from build123d import *

# Parameters (mm, degrees)
ESBO_O2_R                  = 2.8
CORTE_EXTRUS_O1_DEPTH      = 10
CORTE_EXTRUS_O1_DEPTH_BACK = 10
RESSALTO_EXTRUS_O1_START   = -12
ESBO_O5_W                  = 5.6
ESBO_O5_H                  = 16
RESSALTO_EXTRUS_O1_DEPTH   = 80
FILETE1_R                  = 5
CORTE_EXTRUS_O2_DEPTH      = 19


with BuildPart() as part:
    # Esbo_o2 → Revolu_o1 (revolve)
    with BuildSketch(Plane(origin=(0, 0, 0), x_dir=(1, 0, 0), z_dir=(0, 1, 0))):
        with Locations((13.75, 0)):
            Circle(ESBO_O2_R)
    revolve(axis=Axis((0, 0, 0), (0, 0, -1)))

    # Esbo_o3 → Corte-extrus_o1 (cut, two sides)
    with BuildSketch(Plane.XY) as corte_extrus_o1_sk:
        Polygon((-1.202746457, 0), (18.876681975, 24.24777346), (18.876681975, -24.24777346), align=None)
    extrude(amount=CORTE_EXTRUS_O1_DEPTH, mode=Mode.SUBTRACT)
    extrude(corte_extrus_o1_sk.sketch, amount=-CORTE_EXTRUS_O1_DEPTH_BACK, mode=Mode.SUBTRACT)

    # Esbo_o5 → Ressalto-extrus_o1 (add)
    with BuildSketch(Plane(origin=(0, 0, 0), x_dir=(0, 0, -1), z_dir=(1, 0, 0)).offset(RESSALTO_EXTRUS_O1_START)):
        Rectangle(ESBO_O5_W, ESBO_O5_H)
    extrude(amount=-RESSALTO_EXTRUS_O1_DEPTH)

    # Filete1
    filete1_edges = [part.edges().sort_by_distance(p)[0] for p in [
        (-92, -8, 0),
        (-92, 8, 0),
    ]]
    fillet(filete1_edges, radius=FILETE1_R)

    # Esbo_o7 → Corte-extrus_o2 (cut)
    with BuildSketch(Plane(origin=(0, 0, -2.8), x_dir=(-1, 0, 0), z_dir=(0, 0, -1))):
        with BuildLine():
            Line((33.254278711, 4), (83.254278711, 4))
            ThreePointArc((83.254278711, 4), (87.254278711, 0), (83.254278711, -4))
            Line((83.254278711, -4), (33.254278711, -4))
            ThreePointArc((33.254278711, -4), (29.254278711, 0), (33.254278711, 4))
        make_face()
    extrude(amount=-CORTE_EXTRUS_O2_DEPTH, mode=Mode.SUBTRACT)


solid = part.part
Check sheet for the modelled part. Datum: model origin and axes. Units: mm. A direction names the side the tool comes from. Round coordinates to 2 decimals unless told otherwise and drop trailing zeros. Loops run counter-clockwise (first coordinate to the right, second up) from the corner with the lowest first, then second, coordinate; pieces in that order, holes last. Notation, with made-up numbers: (-1.75, 59.5) - (41.25, 59.5) arc R24 cw to (41.25, 70.5) - close; hole circle Ø4 at (66.25, -28.5). An arc over 180 degrees is marked (long way). Answer as CSV lines item,"result". Start each with the question number.
Item 1: Section check A-A (y = 0). Record the boundary of the cut face in (x, z), and give its area (3 significant figures).
Item 2: Depth check by flat-ended pin: P1, Ø1, axis at x = -77.5, z = 0, coming from the +Y side; P2, Ø2, axis at y = -7.5, z = -1.5, coming from the +X side; P3, Ø0.5, axis at y = -2, z = 2.5, coming from the +X side. Enter the tip coordinate at first touch or a pass-through.
Item 3: Set-up check for faces 5 (the cylindrical face through (-90, 7, 0)), 6 (the flat face through (-58, 4, 0)), 7 (the flat face through (8.01, 11.126, -0.039)): record each of +Z, -Z, +X, -X, +Y, -Y from which the full face is reachable in a straight line by a thin tool's end or side.
Item 4: Release check for a two-part mould opening along X. For faces 1 (the cylindrical face through (-87.253, 0.088, -0.039)), 2 (the flat face through (-51, -5, -2.8)), 3 (the cylindrical face through (-91, -6, 0)), 4 (the cylindrical face through (-29.255, -0.088, -0.039)) record: +X half, -X half, draft (parallel to the pull), parting line (faces both ways), or undercut.
Item 5: Scan lines: line 1 (Y direction, x = -79.5, z = -2.1); line 2 (Y direction, x = -14.5, z = 0.95); line 3 (Y direction, x = -32.5, z = 1.6). Record each from-to range of solid material in increasing order. Write a range as [from, to].
Report:
1,outline,"(-92, -2.8) - (-87.25, -2.8) - (-87.25, 2.8) - (-92, 2.8) - close; (-29.25, -2.8) - (-12, -2.8) - (-12, -2.19) arc R2.8 ccw to (-12, 2.19) - (-12, 2.8) - (-29.25, 2.8) - close"
1,area,"126 mm2"
2,P1,"stops at y = 8"
2,P2,"stops at x = -7.35"
2,P3,"stops at x = -11.91"
3,face 5,"+Z, -Z, -X, +Y"
3,face 6,"+Z, -Z"
3,face 7,"+Z, -Z, +X"
4,face 1,"undercut"
4,face 2,"draft"
4,face 3,"-X half"
4,face 4,"undercut"
5,line 1,"y = [-8, -4], [4, 8]"
5,line 2,"y = [-8, 8]"
5,line 3,"y = [-8, -3.93], [3.93, 8]"
